Source: CAD feature listing. Evaluate the final solid. Frame: model axes, mm. A direction names the side the tool comes from. Coordinates: 2 decimals unless noted, no trailing zeros. Loops run counter-clockwise (first coordinate to the right, second up) from the corner with the lowest first, then second, coordinate; pieces in that order, holes last.
Item 1: Pin query (flat end, axial travel): pin 1 Ø3 at (x, z) = (27.5, 4) entering from -Y; pin 2 Ø8 at (y, z) = (-4.5, -5.5) entering from +X; pin 3 Ø4 at (x, z) = (32.5, 1) entering from +Y; pin 4 Ø1 at (x, y) = (10, 3.5) entering from -Z. Return the tip coordinate at first contact, or that it passes through.
Item 2: Section query B-B, the plane x = 21.5. Return the cut outline in (y, z), then the cut area to 3 significant figures.
Item 3: Reachability of faces 1 (the conical face through (0.17, -4.13, 7.19)), 2 (the flat face through (6.85, -4, 3.4)) from +Z, -Z, +X, -X, +Y, -Y: full face, straight path, thin tool, end or side. Return the list, or none.
Item 4: Line query: probe 1 along X at (y, z) = (-6.25, 0.25); probe 2 along Y at (x, z) = (20.5, -0.25); probe 3 along Y at (x, z) = (18, -3). Output: solid intervals per line, ascending.
Item 5: Section query A-A, the plane x = 6. Return the cut outline in (y, z).
```python
from build123d import *

# Parameters (mm, degrees)
BASEHEAD_DEPTH = 6.85


# Read off the part's stored shape, not the designer's step: HeadChamfer
with BuildPart() as part:
    # Sketch1 → BaseHead (new body)
    with BuildSketch(Plane(origin=(0, 0, 0), x_dir=(0, 0, -1), z_dir=(1, 0, 0))):
        Polygon((8, 4.618802154), (8, -4.618802154), (0, -9.237604307), (-8, -4.618802154), (-8, 4.618802154), (0, 9.237604307), align=None)
    extrude(amount=BASEHEAD_DEPTH)

    # HeadChamfer outline → HeadChamfer (revolve, cut)
    with BuildSketch(Plane.YX):
        Polygon((9.237604311, 0.714531182), (8, 0), (9.237604311, 0), align=None)
    revolve(axis=Axis((0, 0, 0), (1, 0, 0)), mode=Mode.SUBTRACT)

    # HeadChamfer 2 outline → HeadChamfer 2 (revolve)
    with BuildSketch(Plane.YX):
        Polygon((5, 6.85), (5, 36.022), (4.172, 36.85), (0, 36.85), (0, 6.85), align=None)
    revolve(axis=Axis((0, 0, 0), (1, 0, 0)))


solid = part.part
```
Verdict:
1. pin 1: stops at y = -4.33
1. pin 2: stops at x = 36.85
1. pin 3: stops at y = 5
1. pin 4: stops at z = -4
2. outline: circle Ø10 at (0, 0)
2. area: 78.5 mm2
3. face 1: +Z, -X, -Y
3. face 2: +X
4. probe 1: x = 0 to 6.85
4. probe 2: y = -4.99 to 4.99
4. probe 3: y = -4 to 4
5. outline: (-9.24, 0) - (-4.62, -8) - (4.62, -8) - (9.24, 0) - (4.62, 8) - (-4.62, 8) - close
